Input: part model. Units: mm. Frame: model coordinates. Coordinates: 2 decimals unless noted, no trailing zeros. Order: outer loops, then holes, each group sorted by start corner. A loop starts at its lowest first (then second) coordinate and runs counter-clockwise, first axis right, second up. Notation, with made-up numbers: M 65,11 L 74,11 A15 cw 74,36 Z; hole C -30.75,67.5 d5. An arc over 180 degrees is marked long. One line per item, written item: value.
```python
from build123d import *

# Parameters (mm, degrees)
SKETCH1_W               = 152.4
SKETCH1_H               = 152.4
BOSS_EXTRUDE1_DEPTH     = 6.35
SKETCH2_W               = 6.35
SKETCH2_H               = 50.8
SKETCH2_W_2             = 50.8
SKETCH2_H_2             = 6.35
CUT_EXTRUDE1_DEPTH      = 6.35
CUT_EXTRUDE1_DEPTH_BACK = 16.51


with BuildPart() as part:
    # Sketch1 → Boss-Extrude1 (new body)
    with BuildSketch(Plane(origin=(0, 0, 0), x_dir=(1, 0, 0), z_dir=(0, 1, 0))):
        with Locations((76.2, 76.2)):
            Rectangle(SKETCH1_W, SKETCH1_H)
    extrude(amount=BOSS_EXTRUDE1_DEPTH)

    # Sketch2 → Cut-Extrude1 (cut, two sides)
    with BuildSketch(Plane(origin=(0, 6.35, 0), x_dir=(1, 0, 0), z_dir=(0, 1, 0))) as cut_extrude1_sk:
        with Locations((9.525, 76.2)):
            Rectangle(SKETCH2_W, SKETCH2_H)
        with Locations((142.875, 76.2)):
            Rectangle(SKETCH2_W, SKETCH2_H)
        with Locations((76.2, 9.525)):
            Rectangle(SKETCH2_W_2, SKETCH2_H_2)
        with Locations((76.2, 142.875)):
            Rectangle(SKETCH2_W_2, SKETCH2_H_2)
    extrude(amount=CUT_EXTRUDE1_DEPTH, mode=Mode.SUBTRACT)
    extrude(cut_extrude1_sk.sketch, amount=-CUT_EXTRUDE1_DEPTH_BACK, mode=Mode.SUBTRACT)


solid = part.part
```
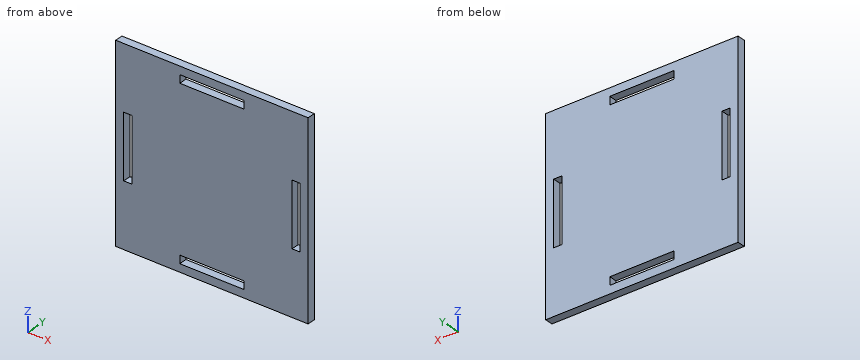
(1) Ray query, line 1 (X direction, y = 5, z = -99); line 2 (Z direction, x = 73, y = 4.25); line 3 (X direction, y = 3, z = -143). Return the intervals inside material, ascending. Write a range as from..to.
Data:
line 1: x = 0..6.35, 12.7..139.7, 146.05..152.4
line 2: z = -152.4..-146.05, -139.7..-12.7, -6.35..0
line 3: x = 0..50.8, 101.6..152.4
(2) Cut plane C-C on y = 5.25. Output: boundary loops of the cut face in (x, z), plus the area to 3 significant figures.
Data:
outline: M 0,-152.4 L 152.4,-152.4 L 152.4,0 L 0,0 Z; hole M 6.35,-101.6 L 12.7,-101.6 L 12.7,-50.8 L 6.35,-50.8 Z; hole M 50.8,-146.05 L 101.6,-146.05 L 101.6,-139.7 L 50.8,-139.7 Z; hole M 50.8,-12.7 L 101.6,-12.7 L 101.6,-6.35 L 50.8,-6.35 Z; hole M 139.7,-101.6 L 146.05,-101.6 L 146.05,-50.8 L 139.7,-50.8 Z
area: 21,900 mm2
(3) Cut plane B-B on x = 87. Output: boundary loops of the cut face in (y, z), plus the area to 3 significant figures.
Data:
outline: M 0,-152.4 L 6.35,-152.4 L 6.35,-146.05 L 0,-146.05 Z; M 0,-139.7 L 6.35,-139.7 L 6.35,-12.7 L 0,-12.7 Z; M 0,-6.35 L 6.35,-6.35 L 6.35,0 L 0,0 Z
area: 887 mm2
(4) Cut plane A-A on z = -55.5. Output: boundary loops of the cut face in (x, y), plus the area to 3 significant figures.
Data:
outline: M 0,0 L 6.35,0 L 6.35,6.35 L 0,6.35 Z; M 12.7,0 L 139.7,0 L 139.7,6.35 L 12.7,6.35 Z; M 146.05,0 L 152.4,0 L 152.4,6.35 L 146.05,6.35 Z
area: 887 mm2
